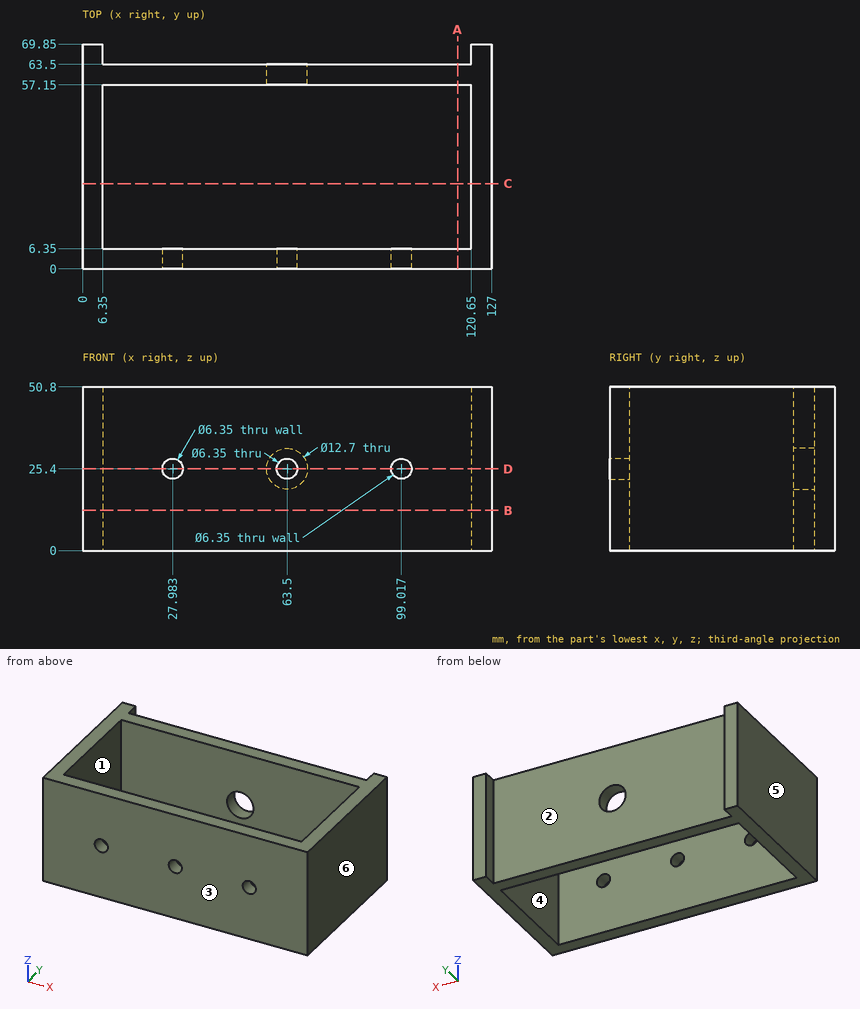
Geometry: see drawing. Coordinates: mm, zero at the bounding-box minimum. A direction names the side the tool comes from. Give positions to 0.01 mm unless a question says otherwise; leave off trailing zeros. Write each loop counter-clockwise with the first axis right and the second up, starting at its lowest first coordinate (ties: lowest second). Pieces come first, ordered by that corner, then holes. Notation, with made-up numbers: M 3.5,-1.75 L 35.5,-1.75 A30 cw 35.5,23.25 Z; hole C -34,-7.75 d3. An arc over 180 degrees is marked long. Answer in a Markdown table with one row per item. Add a question column.
(1) First-contact query: pin 1 (10 mm diameter, centred on x = 99.02, z = 25.4, fed in from +Y); pin 2 (7.5 mm diameter, centred on x = 63.5, z = 25.4, fed in from +Y). Flat tips, straight axial feed; report the tip coordinate or a pass-through.
(2) Section B-B on z = 12.5. Return loops of the section in (x, y), and give its area (3 significant figures).
(3) Ray query, line 1 (X direction, y = 61, z = 25); line 2 (Y direction, x = 44, z = 18); line 3 (X direction, y = 19.5, z = 20). Return the intervals inside material, ascending.
(4) Reachability of the marked faces 1, 2 and 3 from +Z, -Z, +X, -X, +Y, -Y: full face, straight path, thin tool, end or side. Return the list, or none.
(5) Section C-C on y = 26.5. Return loops of the section in (x, z), and give its area (3 significant figures).
(6) Section A-A on x = 116.5. Return loops of the section in (y, z).
(7) Section D-D on z = 25.4. State how many separate pieces and enclosed holes the cut face has, and give its area (3 significant figures).
(8) Mould query, pull axis X, two halves, no side actions, for the marked faces 4, 5 and 6. Classes: +X half, -X half, draft (parallel to the pull), parting line (faces both ways), or undercut.
Result set:
| question | item | result |
|---|---|---|
| 1 | pin 1 | stops at y = 63.5 |
| 1 | pin 2 | stops at y = 6.35 |
| 2 | outline | M 0,0 L 127,0 L 127,69.85 L 120.65,69.85 L 120.65,63.5 L 6.35,63.5 L 6.35,69.85 L 0,69.85 Z; hole M 6.35,6.35 L 120.65,6.35 L 120.65,57.15 L 6.35,57.15 Z |
| 2 | area | 2,340 mm^2 |
| 3 | line 1 | x = 0 to 57.16, 69.84 to 127 |
| 3 | line 2 | y = 0 to 6.35, 57.15 to 63.5 |
| 3 | line 3 | x = 0 to 6.35, 120.65 to 127 |
| 4 | face 1 | +Z, -Z |
| 4 | face 2 | +Z, -Z, +Y |
| 4 | face 3 | +Z, -Z, +X, -X, -Y |
| 5 | outline | M 0,0 L 6.35,0 L 6.35,50.8 L 0,50.8 Z; M 120.65,0 L 127,0 L 127,50.8 L 120.65,50.8 Z |
| 5 | area | 645 mm^2 |
| 6 | outline | M 0,0 L 6.35,0 L 6.35,50.8 L 0,50.8 Z; M 57.15,0 L 63.5,0 L 63.5,50.8 L 57.15,50.8 Z |
| 7 | separate pieces | 4 |
| 7 | enclosed holes | 0 |
| 7 | area | 2,140 mm^2 |
| 8 | face 4 | undercut |
| 8 | face 5 | -X half |
| 8 | face 6 | +X half |
